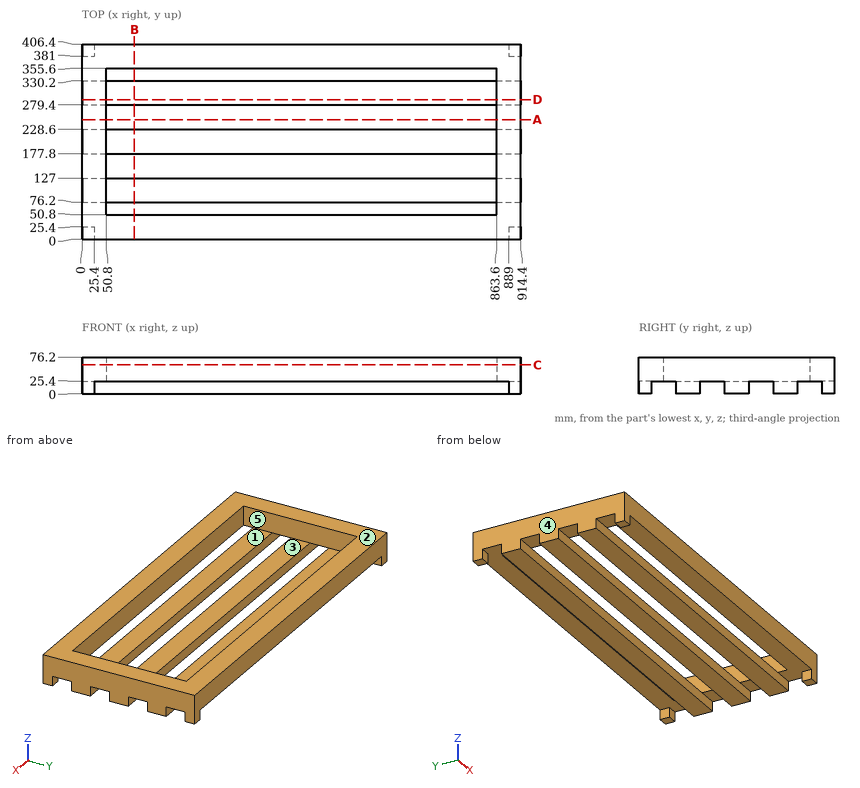
Job drawing, mm, ordinate dimensions from the low corner. One solid piece. A direction names the side the tool comes from. Round coordinates to 2 decimals unless told otherwise and drop trailing zeros. Loops run counter-clockwise (first coordinate to the right, second up) from the corner with the lowest first, then second, coordinate; pieces in that order, holes last. Notation, with made-up numbers: (43, -32) -> (85, -32) arc R16 cw to (85, -16) -> close; hole circle Ø1 at (75.5, 80.5). An arc over 180 degrees is marked (long way). Use CSV: the item, a comma, the result in double quotes. Start each with the question number.
Q1. Flat gauge pins, fed straight in: pin 1 Ø15 at (x, y) = (611, 90) entering from +Z; pin 2 Ø4 at (x, z) = (124, 21.5) entering from -Y; pin 3 Ø15 at (x, y) = (16, 150.5) entering from -Z. Where does each tip first touch, or does it go through?
Q2. Mould opens along Y. For the marked faces 1, 2 and 3 say: +Y half, -Y half, draft (parallel to the pull), parting line (faces both ways), or undercut.
Q3. Which spindle directions (+Z, -Z, +X, -X, +Y, -Y) get a long thin tool onto all of the face, cutting with end or side? Do the marked faces 4 and 5. Say none if no direction does.
Q4. Drill centre lines: L1, parallel to Y at x = 530.5, z = 22; L2, parallel to Y at x = 463, z = 61.5; L3, parallel to X at y = 69.5, z = 53. Where is each one in solid material? Low to high.
Q5. Saw through at D-D on y = 290.5. Give the cut face in (x, z), and give its area (3 significant figures).
Q6. Saw through at A-A on y = 249. Give the cut face in (x, z), and give its area (3 significant figures).
Q7. Saw through at C-C on z = 60. Give the cut face in (x, y), and give its area (3 significant figures).
Q8. Saw through at B-B on x = 109. Give the cut face in (y, z).
Solutions:
1,pin 1,"stops at z = 25.4"
1,pin 2,"stops at y = 76.2"
1,pin 3,"stops at z = 25.4"
2,face 1,"undercut"
2,face 2,"draft"
2,face 3,"undercut"
3,face 4,"+Z, -Z, -X, +Y, -Y"
3,face 5,"+Z"
4,L1,"y = 76.2 to 127, 177.8 to 228.6, 279.4 to 330.2"
4,L2,"y = 0 to 50.8, 355.6 to 406.4"
4,L3,"x = 0 to 50.8, 863.6 to 914.4"
5,outline,"(0, 0) -> (914.4, 0) -> (914.4, 76.2) -> (863.6, 76.2) -> (863.6, 25.4) -> (50.8, 25.4) -> (50.8, 76.2) -> (0, 76.2) -> close"
5,area,"28,400 mm^2"
6,outline,"(0, 25.4) -> (50.8, 25.4) -> (50.8, 76.2) -> (0, 76.2) -> close; (863.6, 25.4) -> (914.4, 25.4) -> (914.4, 76.2) -> (863.6, 76.2) -> close"
6,area,"5,160 mm^2"
7,outline,"(0, 0) -> (914.4, 0) -> (914.4, 406.4) -> (0, 406.4) -> close; hole (50.8, 50.8) -> (863.6, 50.8) -> (863.6, 355.6) -> (50.8, 355.6) -> close"
7,area,"124,000 mm^2"
8,outline,"(0, 25.4) -> (50.8, 25.4) -> (50.8, 76.2) -> (0, 76.2) -> close; (76.2, 0) -> (127, 0) -> (127, 25.4) -> (76.2, 25.4) -> close; (177.8, 0) -> (228.6, 0) -> (228.6, 25.4) -> (177.8, 25.4) -> close; (279.4, 0) -> (330.2, 0) -> (330.2, 25.4) -> (279.4, 25.4) -> close; (355.6, 25.4) -> (406.4, 25.4) -> (406.4, 76.2) -> (355.6, 76.2) -> close"
